Build history of the part. All positions in model axes, mm. A direction names the side the tool comes from. Round coordinates to 2 decimals unless told otherwise and drop trailing zeros. Write each loop counter-clockwise with the first axis right and the second up, starting at its lowest first coordinate (ties: lowest second). Pieces come first, ordered by that corner, then holes. Notation, with made-up numbers: (61.5, -28.75) -> (98.5, -28.75) arc R22 cw to (98.5, -5.75) -> close; hole circle Ø10 at (73.5, 24). An arc over 180 degrees is marked (long way). Return JSON: item names as keys, results as strings.
from build123d import *

# Parameters (mm, degrees)
F1_DEPTH = 32
F2_R     = 6.5
F3_DEPTH = 113.001
F4_R     = 5.5
F5_DEPTH = 25
F6_R     = 5.5
F7_DEPTH = 25


with BuildPart() as f1:
    # F0 (on Front) → F1 (new body)
    with BuildSketch(Plane.XZ):
        Polygon((0, 13), (0, 0), (39, 0), (39, 17), (74, 17), (74, 0), (113, 0), (113, 13), (88, 13), (88, 64), (69, 64), (69, 30), (44, 30), (44, 64), (25, 64), (25, 13), align=None)
    extrude(amount=F1_DEPTH)

    # F2 (on Right) → F3 (cut, through all)
    with BuildSketch(Plane.YZ):
        with Locations((-16, 46)):
            Circle(F2_R)
    extrude(amount=F3_DEPTH, mode=Mode.SUBTRACT)

    # F4 (on Top) → F5 (cut)
    with BuildSketch(Plane.XY):
        with Locations((13, -16)):
            Circle(F4_R)
    extrude(amount=F5_DEPTH, mode=Mode.SUBTRACT)

    # F6 (on Top) → F7 (cut)
    with BuildSketch(Plane.XY):
        with Locations((101, -16)):
            Circle(F6_R)
    extrude(amount=F7_DEPTH, mode=Mode.SUBTRACT)


solid = f1.part
Q1. Wall check: L1, parallel to X at y = -16, z = 7.75; L2, parallel to Z at x = 77, y = -16; L3, parallel to Y at x = 33.5, z = 46. Give the ranges that are in metal, low to high.
Verdict:
{"L1": "x = 0 to 7.5, 18.5 to 39, 74 to 95.5, 106.5 to 113", "L2": "z = 0 to 39.5, 52.5 to 64", "L3": "y = -32 to -22.5, -9.5 to 0"}
Q2. Saw through at C-C on x = 101. List the corners of the cut face in (y, z).
Verdict:
{"outline": "(-32, 0) -> (-21.5, 0) -> (-21.5, 13) -> (-32, 13) -> close; (-10.5, 0) -> (0, 0) -> (0, 13) -> (-10.5, 13) -> close"}
Q3. Saw through at A-A on z = 46. List the corners of the cut face in (x, y).
Verdict:
{"outline": "(25, -32) -> (44, -32) -> (44, -22.5) -> (25, -22.5) -> close; (25, -9.5) -> (44, -9.5) -> (44, 0) -> (25, 0) -> close; (69, -32) -> (88, -32) -> (88, -22.5) -> (69, -22.5) -> close; (69, -9.5) -> (88, -9.5) -> (88, 0) -> (69, 0) -> close"}
Q4. Two-plate mould, pull along X, no slides. Class faces 4 (the flat face through (69, -23, 47)), 5 (the flat face through (88, -16, 38)), 6 (the flat face through (19, -16, 0)): +X half, -X half, draft (parallel to the pull), parting line (faces both ways), or undercut.
Verdict:
{"face 4": "undercut", "face 5": "+X half", "face 6": "draft"}
Q5. Saw through at D-D on y = -13. Count the separate pieces of the cut face and the enclosed holes in it, then the cut area to 3 significant figures.
Verdict:
{"separate pieces": "5", "enclosed holes": "0", "area": "2,560 mm²"}
Q6. Pin check, flat tips, straight feed: pin 1 Ø9.5 at (x, y) = (65, -22) entering from -Z; pin 2 Ø3 at (y, z) = (-26, 24) entering from +X; pin 3 Ø9.5 at (y, z) = (-19, 41) entering from -X. Stop position of each tip, or through.
Verdict:
{"pin 1": "stops at z = 17", "pin 2": "stops at x = 88", "pin 3": "stops at x = 25"}
Q7. 3-axis set-ups, long thin cutter, end or side, ignore diameter. For faces 1 (the flat face through (95, -16, 13)), 2 (the flat face through (57, -16, 30)), 3 (the flat face through (25, -16, 39)): which of +Z, -Z, +X, -X, +Y, -Y reach the whole face in a straight line?
Verdict:
{"face 1": "+Z, +X, +Y, -Y", "face 2": "+Z, +Y, -Y", "face 3": "+Z, -X, +Y, -Y"}
Q8. Saw through at B-B on z = 5. List the corners of the cut face in (x, y), then the cut area to 3 significant figures.
Verdict:
{"outline": "(0, -32) -> (39, -32) -> (39, 0) -> (0, 0) -> close; (74, -32) -> (113, -32) -> (113, 0) -> (74, 0) -> close; hole circle Ø11 at (13, -16); hole circle Ø11 at (101, -16)", "area": "2,310 mm²"}
